Input: part model. Units: mm. Frame: model coordinates. Face numbers are marked on the shaded views. A direction names the side the tool comes from. Coordinates: 2 decimals unless noted, no trailing zeros. Order: outer loops, then holes, each group sorted by start corner. A loop starts at its lowest first (then second) coordinate and runs counter-clockwise, first axis right, second up. Notation, with made-up numbers: (58.25, -34) -> (76.25, -34) arc R23 ccw to (76.25, -15) -> close; hole circle Ø2 at (-18, 50). An arc over 180 degrees is marked (long way). One line per question, with ' | ' between items.
Autodesk Inventor part; units mm, degrees
ref_plane "YZ Plane" through (0, 0, 0) normal (1, 0, 0) x (0, 1, 0)
ref_plane "XZ Plane" through (0, 0, 0) normal (0, 1, 0) x (-1, 0, 0)
ref_plane "XY Plane" through (0, 0, 0) normal (0, 0, 1) x (1, 0, 0)
sketch "Sketch1" plane through (0, 0, 0) normal (0, 0, 1) x (1, 0, 0)
  line L0 (57.5, -28.5) -> (-57.5, -28.5)
  line L1 (-57.5, -28.5) -> (-57.5, 28.5)
  line L2 (-57.5, 28.5) -> (57.5, 28.5)
  line L3 (57.5, 28.5) -> (57.5, -28.5)
  line L4 (57.5, -28.5) -> (-57.5, 28.5) construction
  line L5 (-57.5, -28.5) -> (57.5, 28.5) construction
  line L6 (46.5, -16.5) -> (-46.5, -16.5) construction
  line L7 (-46.5, -16.5) -> (-46.5, 16.5) construction
  line L8 (-46.5, 16.5) -> (46.5, 16.5) construction
  line L9 (46.5, 16.5) -> (46.5, -16.5) construction
  line L10 (46.5, -16.5) -> (-46.5, 16.5) construction
  line L11 (-46.5, -16.5) -> (46.5, 16.5) construction
  line L12 (36, -11.5) -> (-36, -11.5) construction
  line L13 (-36, -11.5) -> (-36, 11.5) construction
  line L14 (-36, 11.5) -> (36, 11.5) construction
  line L15 (36, 11.5) -> (36, -11.5) construction
  line L16 (36, -11.5) -> (-36, 11.5) construction
  line L17 (-36, -11.5) -> (36, 11.5) construction
  circle A0 centre (-46.5, 16.5) radius 2.25
  circle A1 centre (-36, 11.5) radius 2.25
  circle A2 centre (-46.5, -16.5) radius 2.25
  circle A3 centre (-36, -11.5) radius 2.25
  circle A4 centre (46.5, -16.5) radius 2.25
  circle A5 centre (36, -11.5) radius 2.25
  circle A6 centre (36, 11.5) radius 2.25
  circle A7 centre (46.5, 16.5) radius 2.25
  point P0 (0, 0)
  dimension "d0" = 115
  dimension "d1" = 57
  dimension "d2" = 93
  dimension "d3" = 33
  dimension "d4" = 72
  dimension "d5" = 23
  dimension "d6" = 4.5
extrude "Extrusion1" add sketch "Sketch1" along normal blind 30
sketch "Sketch2" plane through (0, 0, 0) normal (0, 0, -1) x (-1, 0, 0)
  circle A0 centre (-46.5, 16.5) radius 2.25
  circle A1 centre (-36, 11.5) radius 2.25
  circle A2 centre (-36, -11.5) radius 2.25
  circle A3 centre (-46.5, -16.5) radius 2.25
  circle A4 centre (36, -11.5) radius 2.25
  circle A5 centre (46.5, -16.5) radius 2.25
  circle A6 centre (36, 11.5) radius 2.25
  circle A7 centre (46.5, 16.5) radius 2.25
  line L0 (-57.5, -28.5) -> (57.5, -28.5)
  line L1 (57.5, -28.5) -> (57.5, 28.5)
  line L2 (57.5, 28.5) -> (-57.5, 28.5)
  line L3 (-57.5, 28.5) -> (-57.5, -28.5)
  circle A8 centre (-46.5, 16.5) radius 2.25
  circle A9 centre (-46.5, 16.5) radius 6
  circle A10 centre (-46.5, -16.5) radius 2.25
  circle A11 centre (-46.5, -16.5) radius 6
  circle A12 centre (46.5, -16.5) radius 6
  circle A13 centre (46.5, 16.5) radius 6
  point P0 (0, 0)
  dimension "d9" = 12
extrude "Extrusion2" cut sketch "Sketch2" against normal blind 7 contours A9 | A11 | A12 | A13
sketch "Sketch6" plane through (0, 0, 30) normal (0, 0, 1) x (1, 0, 0)
  line L0 (21.5, -21.5) -> (-21.5, -21.5)
  line L1 (-21.5, -21.5) -> (-21.5, 21.5)
  line L2 (-21.5, 21.5) -> (21.5, 21.5)
  line L3 (21.5, 21.5) -> (21.5, -21.5)
  line L4 (21.5, -21.5) -> (-21.5, 21.5) construction
  line L5 (-21.5, -21.5) -> (21.5, 21.5) construction
  point P0 (0, 0)
  dimension "d27" = 43
  dimension "d28" = 43
extrude "Extrusion5" cut sketch "Sketch6" against normal blind 15
sketch "Sketch7" plane through (0, 0, 0) normal (0, 1, 0) x (-1, 0, 0)
  line L0 (21.5, 30) -> (-21.5, 30)
  line L1 (21.5, 30) -> (21.5, 15)
  line L2 (21.5, 15) -> (-21.5, 15)
  line L3 (-21.5, 30) -> (-21.5, 15)
  line L4 (57.5, 0) -> (-57.5, 0)
  line L5 (57.5, 0) -> (57.5, 30)
  line L6 (-57.5, 30) -> (57.5, 30)
  line L7 (-57.5, 0) -> (-57.5, 30)
  line L8 (57.5, 30) -> (21.5, 30)
  line L9 (21.5, 30) -> (21.5, 15)
  line L10 (21.5, 15) -> (26.5, 15)
  line L11 (26.5, 15) -> (26.5, 25)
  line L12 (26.5, 25) -> (57.5, 25)
  line L13 (57.5, 30) -> (57.5, 25)
  line L14 (57.5, 0) -> (57.5, 30)
  point P0 (0, 0)
  dimension "d31" = 5
  dimension "d32" = 5
extrude "Extrusion6" cut sketch "Sketch7" along normal mid plane 5 contours L6 L5 L12 L11 L10 L1
chamfer "Chamfer2" distance 3 angle 45 6 edges at (-21.5, 12, 30) (0, 21.5, 30) (-21.5, -12, 30) (0, -21.5, 30) (21.5, 0, 30) (-26.5, 0, 25)
fillet "Fillet2" radius 8 4 edges at (-57.5, 28.5, 15) (-57.5, -28.5, 15) (57.5, -28.5, 15) (57.5, 28.5, 15)
properties part number "sujetador guia ejercedor presion"
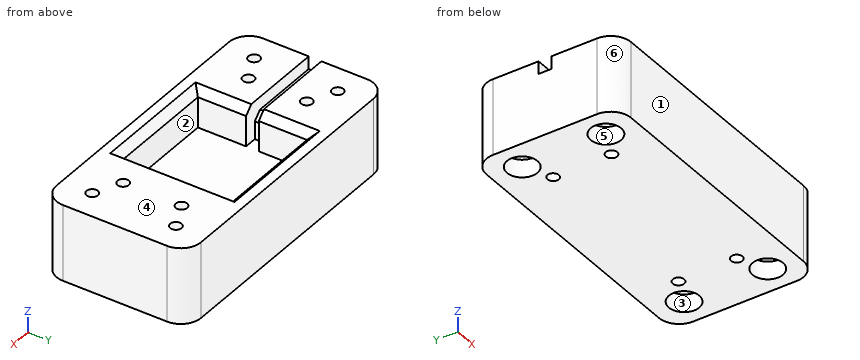
1. Access query for the marked faces 1, 2 and 3. Directions: +Z, -Z, +X, -X, +Y, -Y. A direction counts if a zero-diameter tool reaches every point of the face in a straight line with its end or side. Return the directions, or none.
Recorded:
face 1: +Z, -Z, +X, -X, -Y | face 2: +Z | face 3: -Z
2. Ray query, line 1 (Y direction, x = -36, z = 3.75); line 2 (Y direction, x = 46.5, z = 15); line 3 (X direction, y = -16.5, z = 13.25). Return the intervals inside material, ascending. Write a range as [from, to].
Recorded:
line 1: y = [-28.5, -13.75], [-9.25, 9.25], [13.75, 28.5] | line 2: y = [-28.5, -18.75], [-14.25, 14.25], [18.75, 28.5] | line 3: x = [-57.5, -48.75], [-44.25, 44.25], [48.75, 57.5]
3. Cut plane A-A, the plane x = 36. Return loops of the section in (y, z).
Recorded:
outline: (-28.5, 0) -> (-13.75, 0) -> (-13.75, 30) -> (-28.5, 30) -> close; (-9.25, 0) -> (9.25, 0) -> (9.25, 30) -> (-9.25, 30) -> close; (13.75, 0) -> (28.5, 0) -> (28.5, 30) -> (13.75, 30) -> close
4. Mould query, pull axis X, two halves, no side actions, for the marked faces 4, 5 and 6. Classes: released by +X, released by -X, zero draft, split by the parting line, or undercut.
Recorded:
face 4: zero draft | face 5: undercut | face 6: released by -X
5. Cut plane C-C, the plane z = 3.5. State how many separate pieces and enclosed holes the cut face has, and give its area (3 significant figures).
Recorded:
separate pieces: 1 | enclosed holes: 8 | area: 5,980 mm^2
6. Cut plane D-D, the plane x = -19.5. Return loops of the section in (y, z), and give its area (3 significant figures).
Recorded:
outline: (-28.5, 0) -> (28.5, 0) -> (28.5, 30) -> (24.5, 30) -> (21.5, 27) -> (21.5, 15) -> (-21.5, 15) -> (-21.5, 27) -> (-24.5, 30) -> (-28.5, 30) -> close | area: 1,060 mm^2
7. Cut plane B-B, the plane y = -16.5. Return loops of the section in (x, z), and give its area (3 significant figures).
Recorded:
outline: (-57.5, 0) -> (-52.5, 0) -> (-52.5, 7) -> (-48.75, 7) -> (-48.75, 30) -> (-57.5, 30) -> close; (-44.25, 7) -> (-40.5, 7) -> (-40.5, 0) -> (40.5, 0) -> (40.5, 7) -> (44.25, 7) -> (44.25, 30) -> (24.5, 30) -> (21.5, 27) -> (21.5, 15) -> (-21.5, 15) -> (-21.5, 27) -> (-24.5, 30) -> (-44.25, 30) -> close; (48.75, 7) -> (52.5, 7) -> (52.5, 0) -> (57.5, 0) -> (57.5, 30) -> (48.75, 30) -> close | area: 2,420 mm^2
8. Pin query (flat end, axial travel): pin 1 Ø6 at (x, y) = (-47.5, 17) entering from -Z; pin 2 Ø2.5 at (x, y) = (-50, 1) entering from +Z. Return the tip coordinate at first contact, or that it passes through.
Recorded:
pin 1: stops at z = 7 | pin 2: stops at z = 25
